For this review, take the finished solid that the model builds, in its own axes (mm). Face numbers are marked on the shaded views. A direction names the side the tool comes from. Coordinates: 2 decimals unless noted, no trailing zeros. Loops run counter-clockwise (first coordinate to the right, second up) from the corner with the lowest first, then second, coordinate; pieces in that order, holes last.
1. Take a section at B-B, the plane y = 0. State the section outline as (x, z) points, then the cut area to 3 significant figures.
2. Clearance check with flat-ended pins moving along their axes: P1, Ø2.5, axis at x = -6, y = 0.5, coming from the +Z side; P2, Ø1.5, axis at y = 0, z = 1.5, coming from the -X side; P3, Ø1.6, axis at x = 0, y = 0, coming from the -Z side; P4, Ø1, axis at y = 1, z = -4, coming from the +X side. State where each tip first meets the part, or that it passes through.
3. Machinability: for the marked faces 1 and 2, which of the approach directions +Z, -Z, +X, -X, +Y, -Y give a long, thin tool a straight path to every point of the face, cutting with its end or side? Answer none if there is none.
4. Mouldability with a two-part tool opening along Y and no side actions: class the marked faces 3, 4 and 5 as pulls with the +Y half, pulls with the -Y half, needs draft (parallel to the pull), parting line crosses it, or undercut.
5. Take a section at C-C, the plane x = -7.5. State the section outline as (y, z) points, then the cut area to 3 significant figures.
6. Take a section at D-D, the plane x = -2. State the section outline as (y, z) points, then the cut area to 3 significant figures.
7. Take a section at A-A, the plane z = -4.25. State the section outline as (x, y) points, then the cut area to 3 significant figures.
8. To check wall thickness, follow probe 1 along Z at (x, y) = (-9.25, 1.5); probe 2 along X at (y, z) = (0, -0.5); probe 3 along X at (y, z) = (0, -4). State the ranges of each line that lie inside material, in increasing order.
```python
from build123d import *

# Parameters (mm, degrees)
SKETCH3_R             = 3
SKETCH3_R_2           = 0.9
BOSS_EXTRUDE1_DEPTH   = 12
BOSS_EXTRUDE2_DEPTH   = 6
SKETCH5_W             = 3.2
SKETCH5_H             = 3.2
CUT_EXTRUDE1_DEPTH    = 10
FILLET1_R             = 0.5
CHAMFER1_SIZE         = 0.5
BODY_MOVE_COPY1_ANGLE = 90


with BuildPart() as part:
    # Sketch3 → Boss-Extrude1 (new body)
    with BuildSketch(Plane(origin=(0, 0, 0), x_dir=(1, 0, 0), z_dir=(0, 1, 0))):
        with Locations(Location((0, 0, 0), (0, 0, 270))):
            Circle(SKETCH3_R)
        with Locations(Location((0, 0, 0), (0, 0, 270))):
            Circle(SKETCH3_R_2, mode=Mode.SUBTRACT)
    extrude(amount=BOSS_EXTRUDE1_DEPTH)

    # Boss-Extrude2: read off the stored shape, not the designer's step
    # Boss-Extrude2 outline → Boss-Extrude2 (add)
    with BuildSketch(Plane(origin=(0, 0, 0), x_dir=(1, 0, 0), z_dir=(0, 1, 0))):
        with BuildLine():
            Line((-13, -3), (0, -3))
            ThreePointArc((0, -3), (-3, 0), (0, 3))
            Line((0, 3), (-13, 3))
            Line((-13, 3), (-13, -3))
        make_face()
    extrude(amount=BOSS_EXTRUDE2_DEPTH)

    # Sketch5 → Cut-Extrude1 (cut)
    with BuildSketch(Plane.ZY.offset(13)):
        with Locations((0, 3)):
            Rectangle(SKETCH5_W, SKETCH5_H)
    extrude(amount=-CUT_EXTRUDE1_DEPTH, mode=Mode.SUBTRACT)

    # Fillet1
    # the kernel refuses this fillet: 0.5 mm, written as the material it takes off along each edge
    with BuildSketch(Plane(origin=(-14.25, 0, 3), x_dir=(0, 0, -1), z_dir=(1, 0, 0)), Plane(origin=(0, 0, -3), x_dir=(0, 0, 1), z_dir=(-1, 0, 0))) as fillet1_piece_1:
        with BuildLine():
            CenterArc((FILLET1_R, FILLET1_R), FILLET1_R, 180, 90)
            Line((0, FILLET1_R), (0, 0))
            Line((0, 0), (FILLET1_R, 0))
        make_face()
    extrude(amount=14.25, mode=Mode.SUBTRACT)
    with BuildSketch(Plane(origin=(-14.25, 6, 3), x_dir=(0, 0, -1), z_dir=(1, 0, 0))) as fillet1_piece_2_section:
        with BuildLine():
            CenterArc((FILLET1_R, -FILLET1_R), FILLET1_R, 90, 90)
            Line((0, -FILLET1_R), (0, 0))
            Line((0, 0), (FILLET1_R, 0))
        make_face()
    fillet1_piece_2 = extrude(amount=16.375, mode=Mode.PRIVATE)
    fillet1_piece_2 = fillet1_piece_2 - Plane(origin=(0, 6, 0), x_dir=(0, 0, 1), z_dir=(0, -1, 0)) * Cylinder(3, 35, mode=Mode.PRIVATE)
    add(fillet1_piece_2, mode=Mode.SUBTRACT)
    with BuildSketch(Plane(origin=(2.125, 6, -3), x_dir=(0, -1, 0), z_dir=(-1, 0, 0))) as fillet1_piece_3_section:
        with BuildLine():
            CenterArc((FILLET1_R, FILLET1_R), FILLET1_R, 180, 90)
            Line((0, FILLET1_R), (0, 0))
            Line((0, 0), (FILLET1_R, 0))
        make_face()
    fillet1_piece_3 = extrude(amount=16.375, mode=Mode.PRIVATE)
    fillet1_piece_3 = fillet1_piece_3 - Plane(origin=(0, 6, 0), x_dir=(0, 0, 1), z_dir=(0, -1, 0)) * Cylinder(3, 35, mode=Mode.PRIVATE)
    add(fillet1_piece_3, mode=Mode.SUBTRACT)
    with BuildSketch(Plane(origin=(0, 0, 0), x_dir=(0, 0, 1), z_dir=(-1, 0, 0))) as fillet1_piece_4:
        with BuildLine():
            CenterArc((3 - FILLET1_R, FILLET1_R), FILLET1_R, 270, 90)
            Line((3 - FILLET1_R, 0), (3, 0))
            Line((3, 0), (3, FILLET1_R))
        make_face()
    revolve(axis=Axis((0, 0, 0), (0, 1, 0)), revolution_arc=180, mode=Mode.SUBTRACT)

    # Chamfer1
    chamfer1_edges = [part.edges().sort_by_distance(p)[0] for p in [
        (-13, 3, 1.6),
        (-13, 4.6, 0),
        (-13, 3, -1.6),
        (-13, 1.4, 0),
    ]]
    chamfer(chamfer1_edges, length=CHAMFER1_SIZE)


with BuildPart() as part_1:
    # Body-Move/Copy1: read off the stored shape, not the designer's step
    # Body-Move/Copy1: moved
    add(part.part.moved(Location((0, -6, 0))).rotate(Axis((0, 0, 0), (1, 0, 0)), BODY_MOVE_COPY1_ANGLE))


solid = part_1.part
```
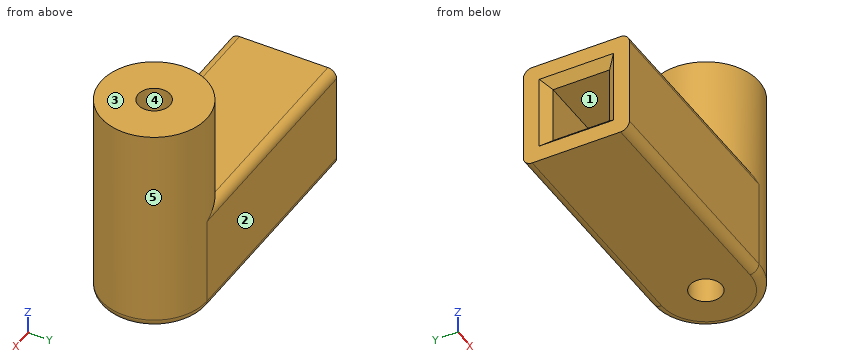
Results list:
1. outline: (-13, -6) - (-0.9, -6) - (-0.9, 6) - (-3, 6) - (-3, 0) - (-13, 0) - (-13, -0.9) - (-12.5, -1.4) - (-3, -1.4) - (-3, -4.6) - (-12.5, -4.6) - (-13, -5.1) - close; (0.9, -6) - (2.5, -6) arc R0.5 ccw to (3, -5.5) - (3, 6) - (0.9, 6) - close
1. area: 78.1 mm2
2. P1: stops at z = 0
2. P2: stops at x = -3
2. P3: passes through
2. P4: stops at x = 2.96
3. face 1: -X
3. face 2: +Z, -Z, +X, -X, +Y
4. face 3: needs draft
4. face 4: undercut
4. face 5: parting line crosses it
5. outline: (-3, -5.5) arc R0.5 ccw to (-2.5, -6) - (2.5, -6) arc R0.5 ccw to (3, -5.5) - (3, -0.5) arc R0.5 ccw to (2.5, 0) - (-2.5, 0) arc R0.5 ccw to (-3, -0.5) - close; hole (-1.6, -4.6) - (1.6, -4.6) - (1.6, -1.4) - (-1.6, -1.4) - close
5. area: 25.5 mm2
6. outline: (-3, -5.5) arc R0.5 ccw to (-2.5, -6) - (2.5, -6) arc R0.5 ccw to (3, -5.5) - (3, -0.5) arc R0.5 ccw to (2.5, 0) - (2.24, 0) - (2.24, 6) - (-2.24, 6) - (-2.24, 0) - (-2.5, 0) arc R0.5 ccw to (-3, -0.5) - close
6. area: 62.6 mm2
7. outline: (-13, -3) - (0, -3) arc R3 ccw to (0, 3) - (-13, 3) - (-13, 2.1) - (-12.5, 1.6) - (-3, 1.6) - (-3, -1.6) - (-12.5, -1.6) - (-13, -2.1) - close; hole circle Ø1.8 at (0, 0)
7. area: 57.3 mm2
8. probe 1: z = -6 to -4.6, -1.4 to 0
8. probe 2: x = -13 to -0.9, 0.9 to 3
8. probe 3: x = -3 to -0.9, 0.9 to 3
